Part print with two shaded views. Sizes in mm from the minimum x, y, z corner. Give positions to 0.01 mm unless a question says otherwise; leave off trailing zeros. Loops run counter-clockwise (first coordinate to the right, second up) from the corner with the lowest first, then second, coordinate; pieces in that order, holes last. Notation, with made-up numbers: (27, -28.75) -> (79, -28.75) arc R23 ccw to (79, -13.75) -> close; hole circle Ø10 at (55.5, -36). An arc over 180 degrees is marked (long way). One line per question, with ' | ' between items. Start each with the question number.
(1) Slice it at B-B, the plane x = 37.5. Write the cut outline in (y, z).
(2) Slice it at C-C, the plane y = 2.55. Give the number of separate pieces and of enclosed holes in the cut face, then the cut area to 3 significant figures.
(3) Flat gauge pins, fed straight in: pin 1 Ø1.6 at (y, z) = (1.5, 47.5) entering from -X; pin 2 Ø0.6 at (y, z) = (2, 9) entering from +X; pin 3 Ø1.6 at (y, z) = (1, 9) entering from -X. Where does each tip first touch, or does it go through?
(4) Drill centre lines: L1, parallel to Z at x = 37.5, y = 1.15; L2, parallel to Z at x = 31.5, y = 1; L3, parallel to X at y = 0.45, z = 23.5 (1 decimal). Where is each one in solid material? Low to high. Write a range as from..to.
(5) Slice it at D-D, the plane x = 49.5. Write the cut outline in (y, z), then the cut area to 3 significant figures.
(6) Slice it at A-A, the plane z = 28. Write the cut outline in (x, y), then the cut area to 3 significant figures.
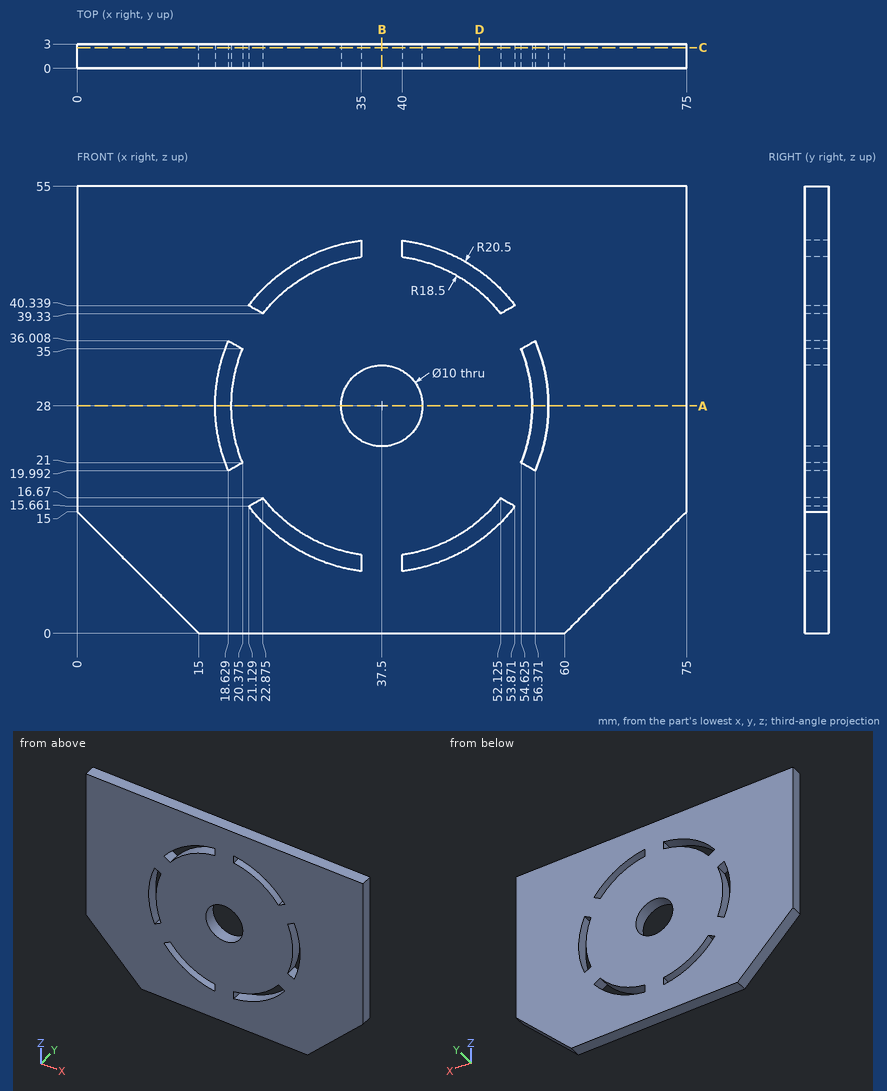
Final values:
1) outline: (0, 0) -> (3, 0) -> (3, 23) -> (0, 23) -> close; (0, 33) -> (3, 33) -> (3, 55) -> (0, 55) -> close
2) separate pieces: 1 | enclosed holes: 7 | area: 3,640 mm2
3) pin 1: x = 0 | pin 2: x = 69.3 | pin 3: x = 5.2
4) L1: 0..23, 33..55 | L2: 0..8.4, 10.5..45.5, 47.6..55 | L3: 0..17.5, 19.6..35.3, 39.7..55.4, 57.5..75
5) outline: (0, 0) -> (3, 0) -> (3, 11.38) -> (0, 11.38) -> close; (0, 13.92) -> (3, 13.92) -> (3, 42.08) -> (0, 42.08) -> close; (0, 44.62) -> (3, 44.62) -> (3, 55) -> (0, 55) -> close | area: 150 mm2
6) outline: (0, 0) -> (17, 0) -> (17, 3) -> (0, 3) -> close; (19, 0) -> (32.5, 0) -> (32.5, 3) -> (19, 3) -> close; (42.5, 0) -> (56, 0) -> (56, 3) -> (42.5, 3) -> close; (58, 0) -> (75, 0) -> (75, 3) -> (58, 3) -> close | area: 183 mm2
